Geometry check sheet. Reference: the model listing, model coordinates, mm. A direction names the side the tool comes from. Coordinates: 2 decimals unless noted, no trailing zeros. Loops run counter-clockwise (first coordinate to the right, second up) from the corner with the lowest first, then second, coordinate; pieces in that order, holes last.
from build123d import *

# Parameters (mm, degrees)
BOSS_EXTRUDE1_DEPTH              = 50.8
F_30_0_1285_DIAMETER_HOLE1_D     = 3.2639
F_30_0_1285_DIAMETER_HOLE2_D     = 3.2639
F_30_0_1285_DIAMETER_HOLE2_DEPTH = 25.4
F_30_0_1285_DIAMETER_HOLE2_TIP   = 0.980574487


with BuildPart() as part:
    # Sketch1 → Boss-Extrude1 (new body)
    with BuildSketch(Plane(origin=(0, 0, 0), x_dir=(1, 0, 0), z_dir=(0, 1, 0))):
        Polygon((0, 0), (31.75, 54.99261314), (34.499630657, 53.40511314), (5.499261314, 3.175), (63.5, 3.175), (63.5, 0), align=None)
    extrude(amount=BOSS_EXTRUDE1_DEPTH)

    # #30 (0.1285) Diameter Hole1 (through all)
    with Locations(Plane.XY):
        with Locations((57.15, 12.7), (57.15, 38.1), (38.1, 38.1), (38.1, 12.7)):
            Hole(F_30_0_1285_DIAMETER_HOLE1_D / 2)

    # #30 (0.1285) Diameter Hole2
    with Locations(Plane(origin=(0, 0, 0), x_dir=(-0.5000000000000039, 0, 0.8660254037844365), z_dir=(-0.8660254037844364, 0, -0.5000000000000038))):
        with Locations((-57.15, 38.1), (-57.15, 12.7), (-38.1, 12.7), (-38.1, 38.1)):
            Hole(F_30_0_1285_DIAMETER_HOLE2_D / 2, depth=F_30_0_1285_DIAMETER_HOLE2_DEPTH)
            with Locations((0, 0, -(F_30_0_1285_DIAMETER_HOLE2_DEPTH + F_30_0_1285_DIAMETER_HOLE2_TIP / 2))):  # 118° drill point
                Cone(0, F_30_0_1285_DIAMETER_HOLE2_D / 2, F_30_0_1285_DIAMETER_HOLE2_TIP, mode=Mode.SUBTRACT)


solid = part.part
(1) Sectioned sample at D-D on z = -11.5. Record the cut outline in (x, y), and give its area (3 significant figures).
Findings:
outline: (6.64, 0) - (10.31, 0) - (10.31, 50.8) - (6.64, 50.8) - close
area: 186 mm2
(2) Draft check along Z on faces 1 (the cylindrical face through (20.82, 11.25, -32.84)), 2 (the cylindrical face through (57.504, 36.507, -1.61)), 3 (the flat face through (33.106, 25.044, -54.21)). Enter one of: +Z half, -Z half, draft (parallel to the pull), parting line (faces both ways), or undercut.
Findings:
face 1: undercut
face 2: draft
face 3: -Z half
(3) Sectioned sample at B-B on x = 25. Record the cut outline in (y, z) (3 decimals).
Findings:
outline: (0, -43.301) - (50.8, -43.301) - (50.8, -36.951) - (0, -36.951) - close; (0, -3.175) - (50.8, -3.175) - (50.8, 0) - (0, 0) - close
(4) Gauge pin test, flat ends, axial feed: pin 1 Ø2 at (y, z) = (9.5, -30.5) entering from +X; pin 2 Ø4 at (y, z) = (44.5, -12.5) entering from -X; pin 3 Ø2 at (x, y) = (57.15, 12.7) entering from +Z; pin 4 Ø1 at (y, z) = (37, -41.5) entering from +X. Record the tip position at first contact, or that the pin passes through.
Findings:
pin 1: stops at x = 21.85
pin 2: stops at x = 6.06
pin 3: passes through
pin 4: stops at x = 27.91
(5) Scan lines: L1, parallel to Y at x = 38, z = -1; L2, parallel to Z at x = 46.5, y = 13.5 (3 decimals); L3, parallel to X at y = 38, z = -2. Record each from-to range of solid material in increasing order.
Findings:
L1: y = 0 to 11.07, 14.33 to 36.47, 39.73 to 50.8
L2: z = -3.175 to 0
L3: x = 1.15 to 36.47, 39.73 to 55.52, 58.78 to 63.5
(6) Access from +Z, -Z, +X, -X, +Y, -Y to the whole of each face (thin tool, end or side, straight path). Record for faces 4 (the flat face through (34, 25, -3.175)), 5 (the flat face through (32, 25, 0)).
Findings:
face 4: +X, +Y, -Y
face 5: +Z, +X, -X, +Y, -Y
(7) Sectioned sample at C-C on y = 38.1. Record the cut outline in (x, z) (3 decimals), and give its area (3 significant figures).
Findings:
outline: (0, 0) - (18.234, -31.582) - (20.984, -29.995) - (5.499, -3.175) - (36.468, -3.175) - (36.468, 0) - close; (19.866, -34.409) - (27.759, -48.08) - (30.509, -46.493) - (22.616, -32.821) - close; (29.391, -50.907) - (31.75, -54.993) - (34.5, -53.405) - (32.141, -49.319) - close; (39.732, -3.175) - (55.518, -3.175) - (55.518, 0) - (39.732, 0) - close; (58.782, -3.175) - (63.5, -3.175) - (63.5, 0) - (58.782, 0) - close
area: 344 mm2
(8) Sectioned sample at A-A on x = 38.1. Record the cut outline in (y, z) (3 decimals), and give its area (3 significant figures).
Findings:
outline: (0, -3.175) - (11.068, -3.175) - (11.068, 0) - (0, 0) - close; (14.332, -3.175) - (36.468, -3.175) - (36.468, 0) - (14.332, 0) - close; (39.732, -3.175) - (50.8, -3.175) - (50.8, 0) - (39.732, 0) - close
area: 141 mm2
